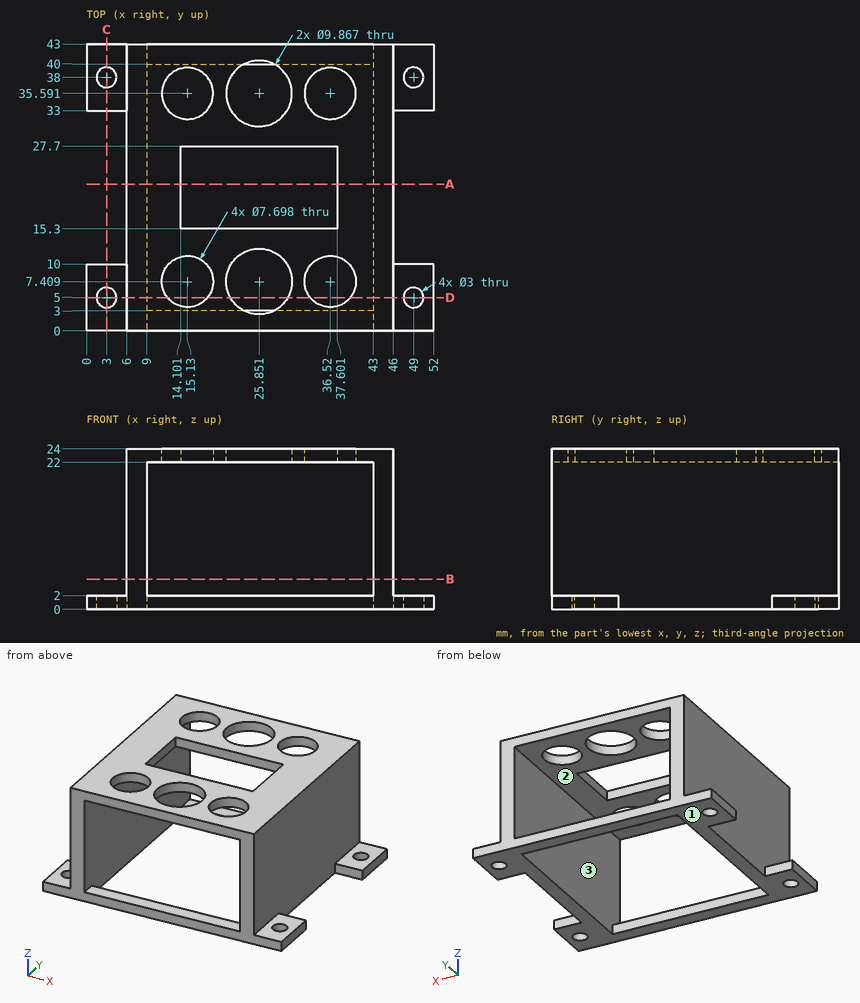
Verification items for this drawing (mm, ordinates from the low corner). Give positions to 0.01 mm unless a question says otherwise; leave off trailing zeros. Loops run counter-clockwise (first coordinate to the right, second up) from the corner with the lowest first, then second, coordinate; pieces in that order, holes last.
(1) Release check for a two-part mould opening along X. For the marked faces 1, 2 and 3 record: released by +X, released by -X, zero draft, split by the parting line, or undercut.
From the geometry:
face 1: zero draft
face 2: undercut
face 3: undercut
(2) Thickness scan on L1, parallel to Y at x = 49, z = 1.4; L2, parallel to Z at x = 36, y = 41.5; L3, parallel to X at y = 17, z = 14.25. Record the ranges inside material, lowest first.
From the geometry:
L1: y = 0 to 3.5, 6.5 to 10, 33 to 36.5, 39.5 to 43
L2: z = 0 to 2, 22 to 24
L3: x = 6 to 9, 43 to 46
(3) Section check D-D on y = 5. Count the separate pieces of the cut face and the enclosed holes in it, then the cut area to 3 significant figures.
From the geometry:
separate pieces: 6
enclosed holes: 0
area: 183 mm2
(4) Depth check by flat-ended pin: pin 1 Ø2 at (x, z) = (48, 1.5) entering from -Y; pin 2 Ø3.5 at (x, y) = (49, 5) entering from +Z; pin 3 Ø6.5 at (y, z) = (29, 14) entering from +X; pin 4 Ø3 at (x, y) = (23.5, 12) entering from -Z. Enter the tip coordinate at first touch or a pass-through.
From the geometry:
pin 1: stops at y = 0
pin 2: stops at z = 2
pin 3: stops at x = 46
pin 4: stops at z = 22
(5) Section check B-B on z = 4.5. Record the cut outline in (x, y).
From the geometry:
outline: (6, 0) - (9, 0) - (9, 43) - (6, 43) - close; (43, 0) - (46, 0) - (46, 43) - (43, 43) - close
(6) Section check A-A on y = 22. Record the cut outline in (x, z).
From the geometry:
outline: (6, 0) - (9, 0) - (9, 22) - (14.1, 22) - (14.1, 24) - (6, 24) - close; (37.6, 22) - (43, 22) - (43, 0) - (46, 0) - (46, 24) - (37.6, 24) - close
(7) Section check C-C on x = 3. Record the cut outline in (y, z), then the cut area to 3 significant figures.
From the geometry:
outline: (0, 0) - (3.5, 0) - (3.5, 2) - (0, 2) - close; (6.5, 0) - (10, 0) - (10, 2) - (6.5, 2) - close; (33, 0) - (36.5, 0) - (36.5, 2) - (33, 2) - close; (39.5, 0) - (43, 0) - (43, 2) - (39.5, 2) - close
area: 28.0 mm2
